For this review, take the finished solid that the model builds, in its own axes (mm). Coordinates: 2 decimals unless noted, no trailing zeros. Write each loop counter-clockwise with the first axis right and the second up, starting at its lowest first coordinate (ties: lowest second). Pieces come first, ordered by that corner, then holes.
1) We need section A-A on y = 20.25. Write out the cut boundary in (x, z), then the cut area to 3 significant figures.
2) We need section C-C on x = 50. Write out the cut boundary in (y, z), then the cut area to 3 significant figures.
3) Insertion check: P1, Ø4, axis at x = 143, z = -7, coming from the +Y side; P2, Ø14, axis at x = 78, y = 21, coming from the +Z side; P3, Ø3, axis at x = 145.5, z = -104.5, coming from the +Y side; P4, Ø11, axis at x = 48.5, z = -101.5, coming from the +Y side. Each pin has a flat end and moves straight along its axis. Give the tip position at first contact, or say it passes through.
4) We need section D-D on z = -48. Write out the cut boundary in (x, y).
5) To check wall thickness, follow line 1 along Z through (x, y) = (143, 0.4); line 2 along X through (y, z) = (1.2, -103); line 3 along X through (y, z) = (10.75, -5). State the ranges of each line that lie inside material, in increasing order.
6) We need section B-B on z = -103. Write out the cut boundary in (x, y), then the cut area to 3 significant figures.
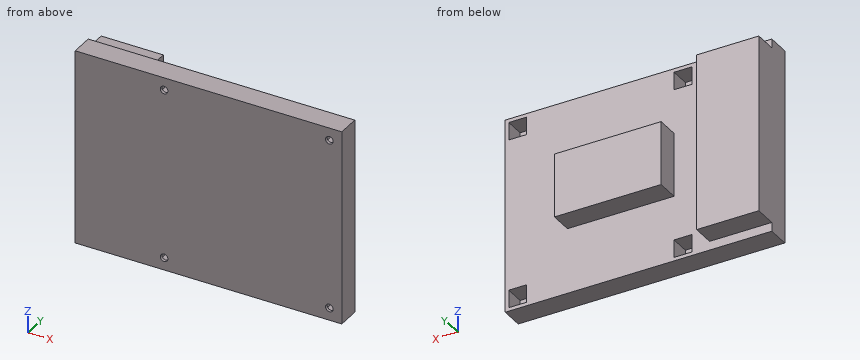
from build123d import *

# Parameters (mm, degrees)
SKETCH1_W                  = 150
SKETCH1_H                  = 110
BOSS_EXTRUDE1_DEPTH        = 1.6
SKETCH2_W                  = 150
SKETCH2_H                  = 110
SKETCH2_W_2                = 10
SKETCH2_H_2                = 10
BOSS_EXTRUDE2_DEPTH        = 11
F_4_0_4_3_DIAMETER_HOLE1_D = 4.3
SKETCH3_W                  = 35
SKETCH3_H                  = 100
BOSS_EXTRUDE3_DEPTH        = 12.6
SKETCH4_W                  = 60
SKETCH4_H                  = 36
BOSS_EXTRUDE4_DEPTH        = 12.6


with BuildPart() as part:
    # Sketch1 → Boss-Extrude1 (new body)
    with BuildSketch(Plane(origin=(0, 0, 0), x_dir=(1, 0, 0), z_dir=(0, 1, 0))):
        with Locations((75, 55)):
            Rectangle(SKETCH1_W, SKETCH1_H)
    extrude(amount=BOSS_EXTRUDE1_DEPTH)

    # Sketch2 → Boss-Extrude2 (add)
    with BuildSketch(Plane(origin=(0, 1.6, 0), x_dir=(1, 0, 0), z_dir=(0, 1, 0))):
        with Locations((75, 55)):
            Rectangle(SKETCH2_W, SKETCH2_H)
        with Locations((50, 103)):
            Rectangle(SKETCH2_W_2, SKETCH2_H_2, mode=Mode.SUBTRACT)
        with Locations((143, 103)):
            Rectangle(SKETCH2_W_2, SKETCH2_H_2, mode=Mode.SUBTRACT)
        with Locations((143, 7)):
            Rectangle(SKETCH2_W_2, SKETCH2_H_2, mode=Mode.SUBTRACT)
        with Locations((50, 7)):
            Rectangle(SKETCH2_W_2, SKETCH2_H_2, mode=Mode.SUBTRACT)
    extrude(amount=BOSS_EXTRUDE2_DEPTH)

    # Ø4.0 (4.3) Diameter Hole1 (through all)
    with Locations(Plane(origin=(0, 1.6, 0), x_dir=(1, 0, 0), z_dir=(0, 1, 0))):
        with Locations((143, 103), (50, 103), (50, 7), (143, 7)):
            Hole(F_4_0_4_3_DIAMETER_HOLE1_D / 2)

    # Sketch3 → Boss-Extrude3 (add)
    with BuildSketch(Plane(origin=(0, 12.6, 0), x_dir=(1, 0, 0), z_dir=(0, 1, 0))):
        with Locations((17.5, 55)):
            Rectangle(SKETCH3_W, SKETCH3_H)
    extrude(amount=BOSS_EXTRUDE3_DEPTH)

    # Sketch4 → Boss-Extrude4 (add)
    with BuildSketch(Plane(origin=(0, 12.6, 0), x_dir=(1, 0, 0), z_dir=(0, 1, 0))):
        with Locations((85, 55)):
            Rectangle(SKETCH4_W, SKETCH4_H)
    extrude(amount=BOSS_EXTRUDE4_DEPTH)


solid = part.part
Result:
1. outline: (0, -105) - (35, -105) - (35, -5) - (0, -5) - close; (55, -73) - (115, -73) - (115, -37) - (55, -37) - close
1. area: 5,660 mm2
2. outline: (0, -110) - (12.6, -110) - (12.6, -108) - (1.6, -108) - (1.6, -105.15) - (0, -105.15) - close; (0, -100.85) - (1.6, -100.85) - (1.6, -98) - (12.6, -98) - (12.6, -12) - (1.6, -12) - (1.6, -9.15) - (0, -9.15) - close; (0, -4.85) - (1.6, -4.85) - (1.6, -2) - (12.6, -2) - (12.6, 0) - (0, 0) - close
2. area: 1,150 mm2
3. P1: passes through
3. P2: stops at z = -37
3. P3: stops at y = 1.6
3. P4: stops at y = 12.6
4. outline: (0, 0) - (150, 0) - (150, 12.6) - (115, 12.6) - (115, 25.2) - (55, 25.2) - (55, 12.6) - (35, 12.6) - (35, 25.2) - (0, 25.2) - close
5. line 1: z = -110 to -105.15, -100.85 to -9.15, -4.85 to 0
5. line 2: x = 0 to 47.85, 52.15 to 140.85, 145.15 to 150
5. line 3: x = 0 to 45, 55 to 138, 148 to 150
6. outline: (0, 0) - (47.85, 0) - (47.85, 1.6) - (45, 1.6) - (45, 12.6) - (35, 12.6) - (35, 25.2) - (0, 25.2) - close; (52.15, 0) - (140.85, 0) - (140.85, 1.6) - (138, 1.6) - (138, 12.6) - (55, 12.6) - (55, 1.6) - (52.15, 1.6) - close; (145.15, 0) - (150, 0) - (150, 12.6) - (148, 12.6) - (148, 1.6) - (145.15, 1.6) - close
6. area: 2,100 mm2
